Input: part model. Units: mm. Frame: model coordinates. A direction names the side the tool comes from. Round coordinates to 2 decimals unless told otherwise and drop trailing zeros. Loops run counter-clockwise (first coordinate to the right, second up) from the corner with the lowest first, then second, coordinate; pieces in that order, holes last. Notation, with made-up numbers: (46, -32.75) - (63, -32.75) arc R35 ccw to (63, 2.25) - close; hole circle Ø10 at (3.25, -12). An arc over 180 degrees is marked (long way). One line per question, with ' | ' between items. Start each with the question number.
Item 1: Section C-C, the plane x = -11. Return loops of the section in (y, z).
Item 2: Material intervals for line 1 along Y through (x, z) = (-18, -0.75); line 2 along Y through (x, z) = (2, -3); line 3 along X through (y, z) = (-47.5, -12), sorted ascending.
Item 3: Set-up query: faces 4 (the face through (-23.717, -25.412, -13.507)), 5 (the face through (23.717, -25.412, -13.507)), 6 (the face through (0, 1, -1)), 7 (the face through (-20.81, -42.95, -13.5)), 8 (the face through (-20.34, -42.84, -7.57)). Return all of +Z, -Z, +X, -X, +Y, -Y with unobstructed straight access to the full face (end or side cutting, diameter ignored); none if empty.
Item 4: First-contact query: pin 1 (2.5 mm diameter, centred on y = -17, z = -10.5, fed in from +X); pin 2 (3.5 mm diameter, centred on x = 20, y = -42.5, fed in from +Z); pin 3 (1 mm diameter, centred on x = -11, y = -17, fed in from +Z). Flat tips, straight axial feed; report the tip coordinate or a pass-through.
Item 5: Draft query along Z for faces 1 (the face through (21, -43, -3)), 2 (the face through (22.06, -37.77, -7.91)), 3 (the face through (30.26, 0.83, -0.49)). Return one class per face: pulls with the +Z half, pulls with the -Z half, needs draft (parallel to the pull), parting line crosses it, or undercut.
Item 6: Section D-D, the plane y = -26. Return loops of the section in (x, z).
Item 7: Section B-B, the plane z = -9. Give the number of separate pieces and of enclosed holes in the cut face, plus the area to 3 significant figures.
Item 8: Section A-A, the plane y = 0. Return loops of the section in (x, z), plus the area to 3 significant figures.
```python
from build123d import *

# Parameters (mm, degrees)
IZIM1_R                         = 2.5
TABAN_FLAN_1_DEPTH              = 1
KENAR_FLAN_1_STRIP_W            = 5.4732
KENAR_FLAN_1_STRIP_H            = 1
KENAR_FLAN_1_STRIP_CUT_DEPTH    = 50
KENAR_FLAN_1_RELIEF_W           = 5.9732
KENAR_FLAN_1_RELIEF_H           = 0.5
KENAR_FLAN_1_RELIEF_CUT_DEPTH   = 1
KENAR_FLAN_1_DEPTH              = 50
KENAR_FLAN_1_START              = 1
KENAR_FLAN_1_FLAT_DEPTH         = 1
KENAR_FLAN_2_STRIP_W            = 5.4732
KENAR_FLAN_2_STRIP_H            = 1
KENAR_FLAN_2_STRIP_CUT_DEPTH    = 16
KENAR_FLAN_2_RELIEF_W           = 5.9732
KENAR_FLAN_2_RELIEF_H           = 0.5
KENAR_FLAN_2_RELIEF_CUT_DEPTH   = 1
KENAR_FLAN_2_STRIP_2_W          = 5.4732
KENAR_FLAN_2_STRIP_2_H          = 1
KENAR_FLAN_2_STRIP_CUT_2_DEPTH  = 16
KENAR_FLAN_2_RELIEF_2_W         = 5.9732
KENAR_FLAN_2_RELIEF_2_H         = 0.5
KENAR_FLAN_2_RELIEF_CUT_2_DEPTH = 1
KENAR_FLAN_2_DEPTH              = 16
KENAR_FLAN_2_BEND_DEPTH         = 16
KES_EKSTR_ZYON1_DEPTH           = 10
KENAR_FLAN_3_DEPTH              = 25
KENAR_FLAN_3_START              = 1
KENAR_FLAN_3_PROFILE_W          = 25
KENAR_FLAN_3_PROFILE_H          = 9.2634
KENAR_FLAN_3_PROFILE_R          = 2
KENAR_FLAN_3_FLAT_DEPTH         = 1
KENAR_FLAN_3_BEND_DEPTH         = 25
KENAR_FLAN_3_PROFILE_2_W        = 25
KENAR_FLAN_3_PROFILE_2_H        = 9.2634
KENAR_FLAN_3_PROFILE_2_R        = 2
KENAR_FLAN_3_FLAT_2_DEPTH       = 1


# Sheet-metal steps are written as plain solids
with BuildPart() as part:
    # Çizim1 → Taban-Flanş1 (new body)
    with BuildSketch(Plane.XY):
        Polygon((-25, 16), (25, 16), (35, 16), (25, -16), (-25, -16), (-35, 16), align=None)
        with Locations((-18, 0)):
            Circle(IZIM1_R, mode=Mode.SUBTRACT)
        with Locations((18, 0)):
            Circle(IZIM1_R, mode=Mode.SUBTRACT)
    extrude(amount=-TABAN_FLAN_1_DEPTH)

    # Kenar-Flanş1 strip (across the edge) → Kenar-Flanş1 strip cut (cut)
    with BuildSketch(Plane(origin=(25, -16, -1), x_dir=(0, 1, 0), z_dir=(-1, 0, 0))):
        with Locations((-2, -0.5)):
            Rectangle(KENAR_FLAN_1_STRIP_W, KENAR_FLAN_1_STRIP_H)
    extrude(amount=KENAR_FLAN_1_STRIP_CUT_DEPTH, mode=Mode.SUBTRACT)

    # Kenar-Flanş1 relief (on the sheet) → Kenar-Flanş1 relief cut (cut)
    with BuildSketch(Plane(origin=(25, -15.2634, -1), x_dir=(0, 1, 0), z_dir=(0, 0, -1))):
        with Locations((-2.4866, 0.25)):
            Rectangle(KENAR_FLAN_1_RELIEF_W, KENAR_FLAN_1_RELIEF_H)
        with Locations((-2.4866, -50.25)):
            Rectangle(KENAR_FLAN_1_RELIEF_W, KENAR_FLAN_1_RELIEF_H)
    extrude(amount=-KENAR_FLAN_1_RELIEF_CUT_DEPTH, mode=Mode.SUBTRACT)

    # Kenar-Flanş1 bend section (across the edge) → Kenar-Flanş1 (add)
    with BuildSketch(Plane(origin=(25, -16, -1), x_dir=(0, 1, 0), z_dir=(-1, 0, 0))):
        with BuildLine():
            Line((-1, 0.7366), (0, 0.7366))
            ThreePointArc((0, 0.7366), (0.215745145, 0.215745145), (0.7366, 0))
            Line((0.7366, 0), (0.7366, -1))
            ThreePointArc((0.7366, -1), (-0.491361636, -0.491361636), (-1, 0.7366))
        make_face()
    extrude(amount=KENAR_FLAN_1_DEPTH)

    # Kenar-Flanş1 profile (on flange) → Kenar-Flanş1 flat (add)
    with BuildSketch(Plane(origin=(0, -16, -1), x_dir=(-1, 0, 0), z_dir=(0, -1, 0)).offset(KENAR_FLAN_1_START)):
        with BuildLine():
            Line((25, 0.7366), (25, 12))
            Line((25, 12), (9, 12))
            ThreePointArc((9, 12), (0, 3), (-9, 12))
            Line((-9, 12), (-25, 12))
            Line((-25, 12), (-25, 0.7366))
            Line((-25, 0.7366), (25, 0.7366))
        make_face()
    extrude(amount=-KENAR_FLAN_1_FLAT_DEPTH)

    # Kenar-Flanş2 strip (across the edge) → Kenar-Flanş2 strip cut (cut)
    with BuildSketch(Plane(origin=(9, -17, -13), x_dir=(0, 0, 1), z_dir=(1, 0, 0))):
        with Locations((-2, -0.5)):
            Rectangle(KENAR_FLAN_2_STRIP_W, KENAR_FLAN_2_STRIP_H)
    extrude(amount=KENAR_FLAN_2_STRIP_CUT_DEPTH, mode=Mode.SUBTRACT)

    # Kenar-Flanş2 relief (on the sheet) → Kenar-Flanş2 relief cut (cut)
    with BuildSketch(Plane(origin=(9, -17, -12.2634), x_dir=(0, 0, 1), z_dir=(0, -1, 0))):
        with Locations((-2.4866, 0.25)):
            Rectangle(KENAR_FLAN_2_RELIEF_W, KENAR_FLAN_2_RELIEF_H)
    extrude(amount=-KENAR_FLAN_2_RELIEF_CUT_DEPTH, mode=Mode.SUBTRACT)

    # Kenar-Flanş2 strip 2 (across the edge) → Kenar-Flanş2 strip cut 2 (cut)
    with BuildSketch(Plane(origin=(-25, -17, -13), x_dir=(0, 0, 1), z_dir=(1, 0, 0))):
        with Locations((-2, -0.5)):
            Rectangle(KENAR_FLAN_2_STRIP_2_W, KENAR_FLAN_2_STRIP_2_H)
    extrude(amount=KENAR_FLAN_2_STRIP_CUT_2_DEPTH, mode=Mode.SUBTRACT)

    # Kenar-Flanş2 relief 2 (on the sheet) → Kenar-Flanş2 relief cut 2 (cut)
    with BuildSketch(Plane(origin=(-25, -17, -12.2634), x_dir=(0, 0, 1), z_dir=(0, -1, 0))):
        with Locations((-2.4866, -16.25)):
            Rectangle(KENAR_FLAN_2_RELIEF_2_W, KENAR_FLAN_2_RELIEF_2_H)
    extrude(amount=-KENAR_FLAN_2_RELIEF_CUT_2_DEPTH, mode=Mode.SUBTRACT)

    # Kenar-Flanş2 section (across the edge) → Kenar-Flanş2 (add)
    with BuildSketch(Plane(origin=(9, -17, -13), x_dir=(0, 0, 1), z_dir=(1, 0, 0))):
        with BuildLine():
            Line((-1, 0.7366), (-1, 38))
            Line((-1, 38), (0, 38))
            Line((0, 38), (0, 0.7366))
            ThreePointArc((0, 0.7366), (0.215745145, 0.215745145), (0.7366, 0))
            Line((0.7366, 0), (0.7366, -1))
            ThreePointArc((0.7366, -1), (-0.491361636, -0.491361636), (-1, 0.7366))
        make_face()
    extrude(amount=KENAR_FLAN_2_DEPTH)

    # Kenar-Flanş2 section 2 (across the edge) → Kenar-Flanş2 bend (add)
    with BuildSketch(Plane(origin=(-25, -17, -13), x_dir=(0, 0, 1), z_dir=(1, 0, 0))):
        with BuildLine():
            Line((-1, 0.7366), (-1, 38))
            Line((-1, 38), (0, 38))
            Line((0, 38), (0, 0.7366))
            ThreePointArc((0, 0.7366), (0.215745145, 0.215745145), (0.7366, 0))
            Line((0.7366, 0), (0.7366, -1))
            ThreePointArc((0.7366, -1), (-0.491361636, -0.491361636), (-1, 0.7366))
        make_face()
    extrude(amount=KENAR_FLAN_2_BEND_DEPTH)

    # Çizim11 → Kes-Ekstrüzyon1 (cut)
    with BuildSketch(Plane(origin=(0, 0, -14), x_dir=(-1, 0, 0), z_dir=(0, 0, -1))):
        Polygon((-16.7, -55), (-25, -20), (-25, -55), align=None)
        Polygon((25, -55), (16.7, -55), (25, -20), align=None)
    extrude(amount=-KES_EKSTR_ZYON1_DEPTH, mode=Mode.SUBTRACT)

    # Kenar-Flanş3 bend section (across the edge) → Kenar-Flanş3 (add)
    with BuildSketch(Plane(origin=(17.41672257, -55.169965638, -13), x_dir=(-0.973014620822144, 0.23074346722353695, 3.4914813388431334e-15), z_dir=(0.23074346722353695, 0.973014620822144, 0))):
        with BuildLine():
            Line((-1, 0.7366), (0, 0.7366))
            ThreePointArc((0, 0.7366), (0.215745145, 0.215745145), (0.7366, 0))
            Line((0.7366, 0), (0.7366, -1))
            ThreePointArc((0.7366, -1), (-0.491361636, -0.491361636), (-1, 0.7366))
        make_face()
    extrude(amount=KENAR_FLAN_3_DEPTH)

    # Kenar-Flanş3 profile (on flange) → Kenar-Flanş3 flat (add)
    with BuildSketch(Plane(origin=(28.875994223, -6.847735773, -13), x_dir=(0.23074346722353695, 0.973014620822144, 0), z_dir=(0.973014620822144, -0.23074346722353695, -3.4914813388431334e-15)).offset(KENAR_FLAN_3_START)):
        with Locations((-37.162388243, 5.3683)):
            Rectangle(KENAR_FLAN_3_PROFILE_W, KENAR_FLAN_3_PROFILE_H)
        with Locations((-44.662388243, 5)):
            Circle(KENAR_FLAN_3_PROFILE_R, mode=Mode.SUBTRACT)
        with Locations((-29.662388243, 5)):
            Circle(KENAR_FLAN_3_PROFILE_R, mode=Mode.SUBTRACT)
    extrude(amount=-KENAR_FLAN_3_FLAT_DEPTH)

    # Kenar-Flanş3 bend section 2 (across the edge) → Kenar-Flanş3 bend (add)
    with BuildSketch(Plane(origin=(-23.18530925, -30.844600117, -13), x_dir=(0.973014620822144, 0.2307434672235371, 3.807964708569791e-15), z_dir=(0.2307434672235371, -0.973014620822144, 0))):
        with BuildLine():
            Line((-1, 0.7366), (0, 0.7366))
            ThreePointArc((0, 0.7366), (0.215745145, 0.215745145), (0.7366, 0))
            Line((0.7366, 0), (0.7366, -1))
            ThreePointArc((0.7366, -1), (-0.491361636, -0.491361636), (-1, 0.7366))
        make_face()
    extrude(amount=KENAR_FLAN_3_BEND_DEPTH)

    # Kenar-Flanş3 profile 2 (on flange) → Kenar-Flanş3 flat 2 (add)
    with BuildSketch(Plane(origin=(-28.875994223, -6.847735773, -13), x_dir=(0.2307434672235371, -0.973014620822144, 0), z_dir=(-0.973014620822144, -0.2307434672235371, -3.807964708569791e-15)).offset(KENAR_FLAN_3_START)):
        with Locations((37.162388243, 5.3683)):
            Rectangle(KENAR_FLAN_3_PROFILE_2_W, KENAR_FLAN_3_PROFILE_2_H)
        with Locations((29.662388243, 5)):
            Circle(KENAR_FLAN_3_PROFILE_2_R, mode=Mode.SUBTRACT)
        with Locations((44.662388243, 5)):
            Circle(KENAR_FLAN_3_PROFILE_2_R, mode=Mode.SUBTRACT)
    extrude(amount=-KENAR_FLAN_3_FLAT_2_DEPTH)


solid = part.part
```
Return value:
1) outline: (-55, -14) - (-17.74, -14) arc R1.74 ccw to (-16, -12.26) - (-16, -1.74) arc R0.74 cw to (-15.26, -1) - (16, -1) - (16, 0) - (-15.26, 0) arc R1.74 ccw to (-17, -1.74) - (-17, -12.26) arc R0.74 cw to (-17.74, -13) - (-55, -13) - close
2) line 1: -16.69 to -2.5, 2.5 to 16 | line 2: -17 to -16 | line 3: -20.26 to -19.24, 19.24 to 20.26
3) face 4: +Z, -Z, -X | face 5: +Z, -Z, +X | face 6: -Z, +X, -X, +Y | face 7: -Z, -X, -Y | face 8: +Z
4) pin 1: x = 25 | pin 2: z = -3 | pin 3: z = -0.52
5) face 1: pulls with the +Z half | face 2: undercut | face 3: needs draft
6) outline: (-23.58, -14) - (-9, -14) - (-9, -13) - (-23.58, -13) - close; (9, -14) - (23.58, -14) - (23.58, -13) - (9, -13) - close
7) separate pieces: 8 | enclosed holes: 0 | area: 70.0 mm2
8) outline: (-30, -1) - (-20.5, -1) - (-20.5, 0) - (-30, 0) - close; (-15.5, -1) - (15.5, -1) - (15.5, 0) - (-15.5, 0) - close; (20.5, -1) - (30, -1) - (30, 0) - (20.5, 0) - close | area: 50.0 mm2
